Here's how the part is built. I have some questions about the finished solid (model axes, mm). Round coordinates to 2 decimals unless told otherwise and drop trailing zeros. Write each loop counter-clockwise with the first axis right and the second up, starting at its lowest first coordinate (ties: lowest second). Pieces come first, ordered by that corner, then holes. Notation, with made-up numbers: M -9.75,-7.5 L -0.75,-7.5 A18 ccw -0.75,21.5 Z; hole C 27,-3.75 d7. An arc over 180 degrees is marked long. Write item = value, one per line. Start each with the question number.
(1) I need wall thicknesses on line 1 along Z through (x, y) = (147.5, -0.6); line 2 along X through (y, z) = (-0.7, 50); line 3 along X through (y, z) = (-0.5, 51). Which ranges of each line are inside material? Lowest first, please.
(2) I want a section at A-A (z = -99.5). List the corners of the cut face in (x, y) for me.
(3) I want a section at B-B (x = 129.5). List the corners of the cut face in (y, z) for me.
(4) I want a section at D-D (x = -151.5). List the corners of the cut face in (y, z) for me.
(5) Will these pins go through, and if not, where does the flat tip stop? pin 1 Ø1 at (y, z) = (-1, -144) entering from +X; pin 2 Ø1 at (y, z) = (-0.5, 161) entering from +X; pin 3 Ø1 at (x, y) = (261, -1) entering from -Z; pin 4 Ø1.9 at (x, z) = (215, 131.5) entering from +Y.
(6) I want a section at C-C (y = -1.3). Give the number of separate pieces and of enclosed holes in the cut face, and give its area (3 significant figures).
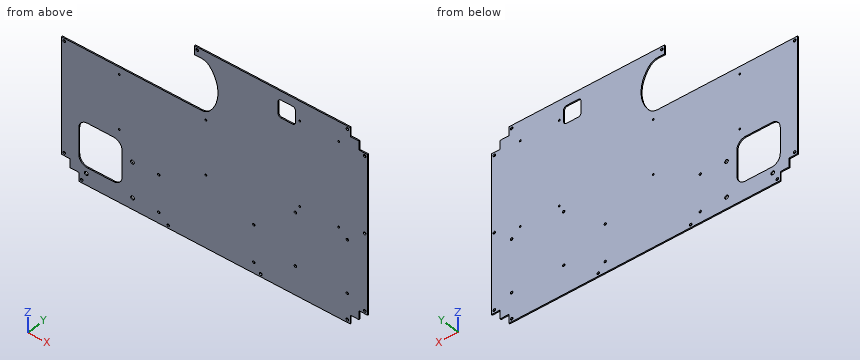
```python
from build123d import *

# Parameters (mm, degrees)
BASE_FLANGE1_DEPTH   = 2
CUT_EXTRUDE1_REACH   = 314.176
CUT_EXTRUDE2_REACH   = 314.176
CUT_EXTRUDE3_REACH   = 314.176
M4_CLEARANCE_HOLE1_D = 4.5
CUT_EXTRUDE4_REACH   = 314.176
SKETCH7_R            = 2
M3_CLEARANCE_HOLE1_D = 3.2
M6_CLEARANCE_HOLE1_D = 6.4
M4_CLEARANCE_HOLE2_D = 4.3


# Sheet-metal steps are written as plain solids
with BuildPart() as part:
    # Sketch1 → Base-Flange1 (new body)
    with BuildSketch(Plane(origin=(0, 0, 0), x_dir=(1, 0, 0), z_dir=(0, 1, 0))):
        Polygon((-250, -150), (-235, -150), (-235, -165), (235, -165), (235, -150), (250, -150), (250, -135), (265, -135), (265, 135), (250, 135), (250, 150), (235, 150), (235, 165), (-235, 165), (-235, 150), (-250, 150), (-250, 135), (-265, 135), (-265, -135), (-250, -135), align=None)
    extrude(amount=-BASE_FLANGE1_DEPTH)

    # Sketch2 → Cut-Extrude1 (cut, up to next)
    with BuildSketch(Plane(origin=(0, 0, 0), x_dir=(1, 0, 0), z_dir=(0, 1, 0)), mode=Mode.PRIVATE) as cut_extrude1_sk1:
        with BuildLine():
            Line((-265, -62.5), (-22.909290949, -62.5))
            ThreePointArc((-22.909290949, -62.5), (-14.653646014, -64.283405184), (-7.870317076, -69.315567329))
            ThreePointArc((-7.870317076, -69.315567329), (6.027337078, -106.25), (-7.870317076, -143.184432671))
            ThreePointArc((-7.870317076, -143.184432671), (-14.653646014, -148.216594816), (-22.909290949, -150))
            Line((-22.909290949, -150), (-35, -150))
            Line((-35, -150), (-35, -165))
            Line((-35, -165), (-265, -165))
            Line((-265, -165), (-265, -62.5))
        make_face()
    cut_extrude1_tool1 = extrude(cut_extrude1_sk1.sketch, amount=-CUT_EXTRUDE1_REACH, mode=Mode.PRIVATE) & part.part
    add(cut_extrude1_tool1.solids().sort_by_distance((-134.940793, 0, 112.899741))[0], mode=Mode.SUBTRACT)

    # Sketch3 → Cut-Extrude2 (cut, up to next)
    with BuildSketch(Plane(origin=(0, 0, 0), x_dir=(1, 0, 0), z_dir=(0, 1, 0)), mode=Mode.PRIVATE) as cut_extrude2_sk1:
        with BuildLine():
            Line((-220, 135), (-175, 135))
            ThreePointArc((-175, 135), (-164.393398282, 130.606601718), (-160, 120))
            Line((-160, 120), (-160, 75))
            ThreePointArc((-160, 75), (-164.393398282, 64.393398282), (-175, 60))
            Line((-175, 60), (-220, 60))
            ThreePointArc((-220, 60), (-230.606601718, 64.393398282), (-235, 75))
            Line((-235, 75), (-235, 120))
            ThreePointArc((-235, 120), (-230.606601718, 130.606601718), (-220, 135))
        make_face()
    cut_extrude2_tool1 = extrude(cut_extrude2_sk1.sketch, amount=-CUT_EXTRUDE2_REACH, mode=Mode.PRIVATE) & part.part
    add(cut_extrude2_tool1.solids().sort_by_distance((-197.5, 0, -97.5))[0], mode=Mode.SUBTRACT)

    # Sketch4 → Cut-Extrude3 (cut, up to next)
    with BuildSketch(Plane(origin=(0, 0, 0), x_dir=(1, 0, 0), z_dir=(0, 1, 0)), mode=Mode.PRIVATE) as cut_extrude3_sk1:
        with BuildLine():
            Line((115, -120), (135, -120))
            ThreePointArc((135, -120), (138.535533906, -121.464466094), (140, -125))
            Line((140, -125), (140, -145))
            ThreePointArc((140, -145), (138.535533906, -148.535533906), (135, -150))
            Line((135, -150), (115, -150))
            ThreePointArc((115, -150), (111.464466094, -148.535533906), (110, -145))
            Line((110, -145), (110, -125))
            ThreePointArc((110, -125), (111.464466094, -121.464466094), (115, -120))
        make_face()
    cut_extrude3_tool1 = extrude(cut_extrude3_sk1.sketch, amount=-CUT_EXTRUDE3_REACH, mode=Mode.PRIVATE) & part.part
    add(cut_extrude3_tool1.solids().sort_by_distance((125, 0, 135))[0], mode=Mode.SUBTRACT)

    # M4 Clearance Hole1 (through all)
    with Locations(Plane(origin=(0, 0, 0), x_dir=(1, 0, 0), z_dir=(0, 1, 0))):
        with Locations((-230, 160), (-80, 160), (80, 160), (230, 160), (260, 130), (260, 0), (260, -130), (230, -160), (-30, -160), (-260, 130), (-260, -57.5)):
            Hole(M4_CLEARANCE_HOLE1_D / 2)

    # Sketch7 → Cut-Extrude4 (cut, up to next)
    with BuildSketch(Plane(origin=(0, 0, 0), x_dir=(1, 0, 0), z_dir=(0, 1, 0)), mode=Mode.PRIVATE) as cut_extrude4_sk1:
        with Locations(Location((-96.5, 146.5, 0), (0, 0, 270))):
            Circle(SKETCH7_R)
    cut_extrude4_tool1 = extrude(cut_extrude4_sk1.sketch, amount=-CUT_EXTRUDE4_REACH, mode=Mode.PRIVATE) & part.part
    # Sketch7 → Cut-Extrude4 (cut, up to next)
    with BuildSketch(Plane(origin=(0, 0, 0), x_dir=(1, 0, 0), z_dir=(0, 1, 0)), mode=Mode.PRIVATE) as cut_extrude4_sk2:
        with Locations(Location((-96.5, 83.5, 0), (0, 0, 270))):
            Circle(SKETCH7_R)
    cut_extrude4_tool2 = extrude(cut_extrude4_sk2.sketch, amount=-CUT_EXTRUDE4_REACH, mode=Mode.PRIVATE) & part.part
    # Sketch7 → Cut-Extrude4 (cut, up to next)
    with BuildSketch(Plane(origin=(0, 0, 0), x_dir=(1, 0, 0), z_dir=(0, 1, 0)), mode=Mode.PRIVATE) as cut_extrude4_sk3:
        with Locations(Location((68, 83.5, 0), (0, 0, 270))):
            Circle(SKETCH7_R)
    cut_extrude4_tool3 = extrude(cut_extrude4_sk3.sketch, amount=-CUT_EXTRUDE4_REACH, mode=Mode.PRIVATE) & part.part
    # Sketch7 → Cut-Extrude4 (cut, up to next)
    with BuildSketch(Plane(origin=(0, 0, 0), x_dir=(1, 0, 0), z_dir=(0, 1, 0)), mode=Mode.PRIVATE) as cut_extrude4_sk4:
        with Locations(Location((68, 146.5, 0), (0, 0, 270))):
            Circle(SKETCH7_R)
    cut_extrude4_tool4 = extrude(cut_extrude4_sk4.sketch, amount=-CUT_EXTRUDE4_REACH, mode=Mode.PRIVATE) & part.part
    add(cut_extrude4_tool1.solids().sort_by_distance((-96.5, 0, -146.5))[0], mode=Mode.SUBTRACT)
    add(cut_extrude4_tool2.solids().sort_by_distance((-96.5, 0, -83.5))[0], mode=Mode.SUBTRACT)
    add(cut_extrude4_tool3.solids().sort_by_distance((68, 0, -83.5))[0], mode=Mode.SUBTRACT)
    add(cut_extrude4_tool4.solids().sort_by_distance((68, 0, -146.5))[0], mode=Mode.SUBTRACT)

    # M3 Clearance Hole1 (through all)
    with Locations(Plane(origin=(0, 0, 0), x_dir=(1, 0, 0), z_dir=(0, 1, 0))):
        with Locations((147.5, 12.5), (215, -131.5), (147.5, -131.5), (215, 12.5), (-15, -50), (-165, 42.5), (-15, 42.5), (-165, -50)):
            Hole(M3_CLEARANCE_HOLE1_D / 2)

    # M6 Clearance Hole1 (through all)
    with Locations(Plane(origin=(0, 0, 0), x_dir=(1, 0, 0), z_dir=(0, 1, 0))):
        with Locations((-142, 145.5), (-222, 145.5), (-142, 85.5)):
            Hole(M6_CLEARANCE_HOLE1_D / 2)

    # M4 Clearance Hole2 (through all)
    with Locations(Plane(origin=(0, 0, 0), x_dir=(1, 0, 0), z_dir=(0, 1, 0))):
        with Locations((230, 116), (140, 26), (230, 26), (140, 116)):
            Hole(M4_CLEARANCE_HOLE2_D / 2)


solid = part.part
```
Returned:
q1.line_1 = -165 to -14.1, -10.9 to 129.9, 133.1 to 165
q1.line_2 = -265 to -166.6, -163.4 to -16.6, -13.4 to 265
q1.line_3 = -265 to -166.25, -163.75 to -16.25, -13.75 to 265
q2.outline = M -265,-2 L -235,-2 L -235,0 L -265,0 Z; M -160,-2 L 265,-2 L 265,0 L -160,0 Z
q3.outline = M -2,-165 L 0,-165 L 0,120 L -2,120 Z; M -2,150 L 0,150 L 0,165 L -2,165 Z
q4.outline = M -2,-165 L 0,-165 L 0,62.5 L -2,62.5 Z
q5.pin_1 = 250
q5.pin_2 = 235
q5.pin_3 = -135
q5.pin_4 = through
q6.separate_pieces = 1
q6.enclosed_holes = 32
q6.area = 140,000 mm²
